Autodesk Inventor part; units mm, degrees
ref_plane "YZ Plane" through (0, 0, 0) normal (1, 0, 0) x (0, 1, 0)
ref_plane "XZ Plane" through (0, 0, 0) normal (0, 1, 0) x (-1, 0, 0)
ref_plane "XY Plane" through (0, 0, 0) normal (0, 0, 1) x (1, 0, 0)
sketch "スケッチ1" plane through (0, 0, 0) normal (0, 0, 1) x (1, 0, 0)
  circle A0 centre (0, 0) radius 1.85
  dimension "d0" = 3.7
extrude "押し出し1" add sketch "スケッチ1" along normal blind 2
sketch "スケッチ2" plane through (0, 0, 0) normal (0, 0, -1) x (-1, 0, 0)
  circle A0 centre (0, 0) radius 1
  dimension "d3" = 2
extrude "押し出し2" add sketch "スケッチ2" along normal blind 6
thread "ねじ1"
chamfer "面取り1" distance 0.2 angle 45 1 edges at (-1.85, 0, 2)
properties part number "M2×6" material "ステンレス鋼"
For this review, take the finished solid that the model builds, in its own axes (mm). A direction names the side the tool comes from. Round coordinates to 2 decimals unless told otherwise and drop trailing zeros. Write each loop counter-clockwise with the first axis right and the second up, starting at its lowest first coordinate (ties: lowest second). Pieces come first, ordered by that corner, then holes. Notation, with made-up numbers: (83.5, -10.75) -> (89.5, -10.75) arc R17 ccw to (89.5, 12.25) -> close; hole circle Ø7 at (34.5, 40). An arc over 180 degrees is marked (long way). One line per question, with ' | ' between items. Start each with the question number.
(1) Tool access review of faces 3 (the face through (0, 0, 2)), 4 (the face through (0, 1, -3)): name each direction out of +Z, -Z, +X, -X, +Y, -Y from which nothing blocks a thin tool from reaching the whole face with its end or side.
(2) Add section A-A, the plane y = 0. Write out the cut boundary in (x, z).
(3) Add section D-D, the plane z = 1.25. Write out the cut boundary in (x, y), plus the area to 3 significant figures.
(4) For line 1 along Z through (x, y) = (-1.3, 0.15); line 2 along Y through (x, z) = (-0.05, -0.5); line 3 along X through (y, z) = (-0.35, 1), list the stretches that pass through material, from the lowest coordinate up. Write a range as from..to.
(5) Insertion check: P1, Ø2, axis at y = -1, z = -4.5, coming from the +X side; P2, Ø1.5, axis at y = -0.5, z = 0.5, coming from the +X side. Each pin has a flat end and moves straight along its axis. Give the tip position at first contact, or say it passes through.
(6) Add section C-C, the plane z = -5.25. Write out the cut boundary in (x, y).
(7) Mouldability with a two-part tool opening along Y and no side actions: class faces 1 (the face through (-0.401, 1.806, 0.887)), 2 (the face through (1, -1, 0)) as released by +Y, released by -Y, zero draft, split by the parting line, or undercut.
Answer list:
1) face 3: +Z, +X, -X, +Y, -Y | face 4: -Z
2) outline: (-1.85, 0) -> (-1, 0) -> (-1, -6) -> (1, -6) -> (1, 0) -> (1.85, 0) -> (1.85, 1.8) -> (1.65, 2) -> (-1.65, 2) -> (-1.85, 1.8) -> close
3) outline: circle Ø3.7 at (0, 0) | area: 10.8 mm²
4) line 1: 0..2 | line 2: -1..1 | line 3: -1.82..1.82
5) P1: x = 1 | P2: x = 1.85
6) outline: circle Ø2 at (0, 0)
7) face 1: split by the parting line | face 2: zero draft
